The model under review builds one solid part; all positions refer to its coordinate system, in mm. A direction names the side the tool comes from. Give positions to 0.01 mm unless a question says otherwise; leave off trailing zeros.
from build123d import *

# Parameters (mm, degrees)
SKETCH1_W           = 185
SKETCH1_H           = 75
BOSS_EXTRUDE1_DEPTH = 58
CUT_EXTRUDE1_DEPTH  = 0.5
CUT_EXTRUDE2_DEPTH  = 0.5
FILLET1_R           = 13
FILLET2_R           = 1


with BuildPart() as part:
    # Sketch1 → Boss-Extrude1 (new body)
    with BuildSketch(Plane(origin=(0, 0, -15), x_dir=(-1, 0, 0), z_dir=(0, 0, -1))):
        with Locations((23.5, 15.5)):
            Rectangle(SKETCH1_W, SKETCH1_H)
    extrude(amount=-BOSS_EXTRUDE1_DEPTH)

    # Sketch2 → Cut-Extrude1 (cut)
    with BuildSketch(Plane(origin=(69, 0, 0), x_dir=(0, 0, -1), z_dir=(1, 0, 0))):
        with BuildLine():
            Line((-34.3, 36.75), (-34.3, -5.75))
            ThreePointArc((-34.3, -5.75), (-32.835533906, -9.285533906), (-29.3, -10.75))
            Line((-29.3, -10.75), (1.3, -10.75))
            ThreePointArc((1.3, -10.75), (4.835533906, -9.285533906), (6.3, -5.75))
            Line((6.3, -5.75), (6.3, 36.75))
            ThreePointArc((6.3, 36.75), (4.835533906, 40.285533906), (1.3, 41.75))
            Line((1.3, 41.75), (-29.3, 41.75))
            ThreePointArc((-29.3, 41.75), (-32.835533906, 40.285533906), (-34.3, 36.75))
        make_face()
    extrude(amount=-CUT_EXTRUDE1_DEPTH, mode=Mode.SUBTRACT)

    # Sketch3 → Cut-Extrude2 (cut)
    with BuildSketch(Plane.ZY.offset(116)):
        with BuildLine():
            Line((27.75, 43.625), (0.25, 43.625))
            ThreePointArc((0.25, 43.625), (-5.406854249, 41.281854249), (-7.75, 35.625))
            Line((-7.75, 35.625), (-7.75, -4.625))
            ThreePointArc((-7.75, -4.625), (-5.406854249, -10.281854249), (0.25, -12.625))
            Line((0.25, -12.625), (27.75, -12.625))
            ThreePointArc((27.75, -12.625), (33.406854249, -10.281854249), (35.75, -4.625))
            Line((35.75, -4.625), (35.75, 35.625))
            ThreePointArc((35.75, 35.625), (33.406854249, 41.281854249), (27.75, 43.625))
        make_face()
    extrude(amount=-CUT_EXTRUDE2_DEPTH, mode=Mode.SUBTRACT)

    # Fillet1
    # the kernel refuses this fillet: 13 mm, written as the material it takes off along each edge
    with BuildSketch(Plane(origin=(-116, -54.5, -15), x_dir=(0, 0, 1), z_dir=(0, 1, 0))) as fillet1_piece_1:
        with BuildLine():
            CenterArc((FILLET1_R, FILLET1_R), FILLET1_R, 180, 90)
            Line((0, FILLET1_R), (0, 0))
            Line((0, 0), (FILLET1_R, 0))
        make_face()
    extrude(amount=140, mode=Mode.SUBTRACT)
    with BuildSketch(Plane(origin=(-116, -54.5, 43), x_dir=(0, 0, -1), z_dir=(0, 1, 0))) as fillet1_piece_2:
        with BuildLine():
            CenterArc((FILLET1_R, -FILLET1_R), FILLET1_R, 90, 90)
            Line((0, -FILLET1_R), (0, 0))
            Line((0, 0), (FILLET1_R, 0))
        make_face()
    extrude(amount=140, mode=Mode.SUBTRACT)

    # Fillet2
    fillet2_edges = [part.edges().sort_by_distance(p)[0] for p in [
        (69, 15.5, 43),
        (-17, -22, -15),
        (69, 15.5, -15),
        (-17, 53, -15),
        (-116, 53, 14),
        (-17, 53, 43),
        (-112.192388155, 53, 39.192388155),
        (-112.192388155, 53, -11.192388155),
        (-116, -22, 14),
        (-17, -22, 43),
        (-112.192388155, -22, 39.192388155),
        (69, 53, 14),
        (-112.192388155, -22, -11.192388155),
        (69, -22, 14),
    ]]
    fillet(fillet2_edges, radius=FILLET2_R)


solid = part.part
1) To check wall thickness, follow probe 1 along X at (y, z) = (12, 13); probe 2 along X at (y, z) = (-8, -8.5); probe 3 along Z at (x, y) = (-106, 2). State the ranges of each line that lie inside material, in increasing order.
2) Tool access review of faces 1 (the cylindrical face through (-110.34, 14.99, -12.73)), 2 (the flat face through (68.5, 16, 14)): name each direction out of +Z, -Z, +X, -X, +Y, -Y from which nothing blocks a thin tool from reaching the whole face with its end or side.
3) The part is to be moulded in two halves that separate along Y. For faces 3 (the flat face through (-116, -17, 14)), 4 (the flat face through (-22, -22, 14)), 5 (the flat face through (-22, 53, 14)), 6 (the cylindrical face through (68.75, -9.32, -4.8)), say which applies: +Y half, -Y half, draft (parallel to the pull), parting line (faces both ways), or undercut.
4) Insertion check: pin 1 (0.6 mm diameter, centred on x = 69, z = 13.5, fed in from -Y); pin 2 (8 mm diameter, centred on y = 36.5, z = 16.5, fed in from -X); pin 3 (12 mm diameter, centred on y = 27, z = -3.5, fed in from +X); pin 4 (1.5 mm diameter, centred on y = 16, z = -7.5, fed in from -X). Each pin has a flat end and moves straight along its axis. Give the tip position at first contact, or say it passes through.
Answer block:
1. probe 1: x = -115.5 to 68.5
1. probe 2: x = -114.26 to 69
1. probe 3: z = -14.65 to 42.65
2. face 1: -Z, -X, +Y, -Y
2. face 2: +X
3. face 3: draft
3. face 4: -Y half
3. face 5: +Y half
3. face 6: undercut
4. pin 1: stops at y = -21.71
4. pin 2: stops at x = -115.5
4. pin 3: stops at x = 69
4. pin 4: stops at x = -115.1
